```python
from build123d import *

# Parameters (mm, degrees)
SKETCH1_W               = 92
SKETCH1_H               = 70
SKETCH1_R               = 14.6
BOSS_EXTRUDE1_DEPTH     = 5
CUT_EXTRUDE1_DEPTH      = 116.71084651
CUT_EXTRUDE1_DEPTH_BACK = 116.71084651
SKETCH2_R               = 2.5
CUT_EXTRUDE2_DEPTH      = 116.71084651
CUT_EXTRUDE2_DEPTH_BACK = 116.71084651
SKETCH3_R               = 3


with BuildPart() as part:
    # Sketch1 → Boss-Extrude1 (new body)
    with BuildSketch(Plane(origin=(0, 0, 0), x_dir=(0, 0, -1), z_dir=(1, 0, 0))):
        with Locations((46, -35)):
            Rectangle(SKETCH1_W, SKETCH1_H)
        with Locations((46, -35)):
            Circle(SKETCH1_R, mode=Mode.SUBTRACT)
    extrude(amount=BOSS_EXTRUDE1_DEPTH)

    # Sketch2 → Cut-Extrude1 (cut, two sides: drawn at the far end of the back side and taken through both)
    with BuildSketch(Plane(origin=(5, 0, 0), x_dir=(0, 0, -1), z_dir=(1, 0, 0)).offset(-CUT_EXTRUDE1_DEPTH_BACK)):
        with Locations((5, -53.727554141)):
            Circle(SKETCH2_R)
        with Locations((5, -16.272445859)):
            Circle(SKETCH2_R)
        with Locations((87, -53.727554141)):
            Circle(SKETCH2_R)
        with Locations((87, -16.272445859)):
            Circle(SKETCH2_R)
    extrude(amount=CUT_EXTRUDE1_DEPTH + CUT_EXTRUDE1_DEPTH_BACK, mode=Mode.SUBTRACT)

    # Sketch3 → Cut-Extrude2 (cut, two sides: drawn at the far end of the back side and taken through both)
    with BuildSketch(Plane.ZY.offset(-CUT_EXTRUDE2_DEPTH_BACK)):
        with Locations((-46, -8.059478057)):
            Circle(SKETCH3_R)
    extrude(amount=CUT_EXTRUDE2_DEPTH + CUT_EXTRUDE2_DEPTH_BACK, mode=Mode.SUBTRACT)


solid = part.part
```
Work out the finished part from the listing and answer in its coordinate system (mm). Round coordinates to 2 decimals unless told otherwise and drop trailing zeros. Write each loop counter-clockwise with the first axis right and the second up, starting at its lowest first coordinate (ties: lowest second). Pieces come first, ordered by that corner, then holes. Notation, with made-up numbers: (-31, 82.25) -> (14, 82.25) arc R8 cw to (14, 86.25) -> close; hole circle Ø5 at (69.5, 12). An arc over 180 degrees is marked (long way). Write each question's results on one line, items separated by ' | '.
Q1. Straight lines are drawn through the part: line 1 along Y through (x, z) = (2.8, -46); line 2 along Y through (x, z) = (3.3, -87); line 3 along Z through (x, y) = (3.1, -16). For each, find the intervals that lie inside material, in ascending order. Write a range as [from, to].
Data:
line 1: [-70, -49.6], [-20.4, -11.06], [-5.06, 0] | line 2: [-70, -56.23], [-51.23, -18.77], [-13.77, 0] | line 3: [-92, -89.49], [-84.51, -7.49], [-2.51, 0]
Q2. Section B-B, the plane z = -5 is taken. Write down the section's boundary in (x, y).
Data:
outline: (0, -70) -> (5, -70) -> (5, -56.23) -> (0, -56.23) -> close; (0, -51.23) -> (5, -51.23) -> (5, -18.77) -> (0, -18.77) -> close; (0, -13.77) -> (5, -13.77) -> (5, 0) -> (0, 0) -> close
Q3. Section C-C, the plane z = -59.5 is taken. Write down the section's boundary in (x, y), then the cut area to 3 significant figures.
Data:
outline: (0, -70) -> (5, -70) -> (5, -40.56) -> (0, -40.56) -> close; (0, -29.44) -> (5, -29.44) -> (5, 0) -> (0, 0) -> close | area: 294 mm^2
Q4. Determine the mould class of faces 1 (the flat face through (5, -50, -45)), 2 (the flat face through (2, -35, -92)), 3 (the cylindrical face through (2.465, -13.794, -4.675)) for opening direction Z: released by +Z, released by -Z, zero draft, split by the parting line, or undercut.
Data:
face 1: zero draft | face 2: released by -Z | face 3: undercut
Q5. Flat-ended cylindrical pins translate along their axes: P1, Ø6, axis at y = -16.27, z = -87, coming from the -X side; P2, Ø3, axis at y = -16.27, z = -5, coming from the +X side. Find the tip coordinate at first contact, or state that the pin passes through.
Data:
P1: x = 0 | P2: through
Q6. Section D-D, the plane x = 2.35 is taken. Write down the section's boundary in (y, z).
Data:
outline: (-70, -92) -> (0, -92) -> (0, 0) -> (-70, 0) -> close; hole circle Ø5 at (-53.73, -87); hole circle Ø5 at (-53.73, -5); hole circle Ø29.2 at (-35, -46); hole circle Ø5 at (-16.27, -87); hole circle Ø5 at (-16.27, -5); hole circle Ø6 at (-8.06, -46)
Q7. Section A-A, the plane y = -35 is taken. Write down the section's boundary in (x, z), then the cut area to 3 significant figures.
Data:
outline: (0, -92) -> (5, -92) -> (5, -60.6) -> (0, -60.6) -> close; (0, -31.4) -> (5, -31.4) -> (5, 0) -> (0, 0) -> close | area: 314 mm^2
